```python
from build123d import *

# Parameters (mm, degrees)
F0_W     = 76
F0_H     = 70
F1_DEPTH = 3
F3_D     = 8.3
F4_SIZE  = 5


with BuildPart() as f1:
    # F0 (on Top) → F1 (new body)
    with BuildSketch(Plane.XY):
        Rectangle(F0_W, F0_H)
    extrude(amount=-F1_DEPTH)

    # F3 (through all)
    with Locations(Plane.XY):
        with Locations((-30, 25), (30, 25), (30, -25), (-30, -25)):
            Hole(F3_D / 2)

    # F4
    f4_edges = [f1.edges().sort_by_distance(p)[0] for p in [
        (-38, 35, -1.5),
        (-38, -35, -1.5),
        (38, -35, -1.5),
        (38, 35, -1.5),
    ]]
    chamfer(f4_edges, length=F4_SIZE)


solid = f1.part
```
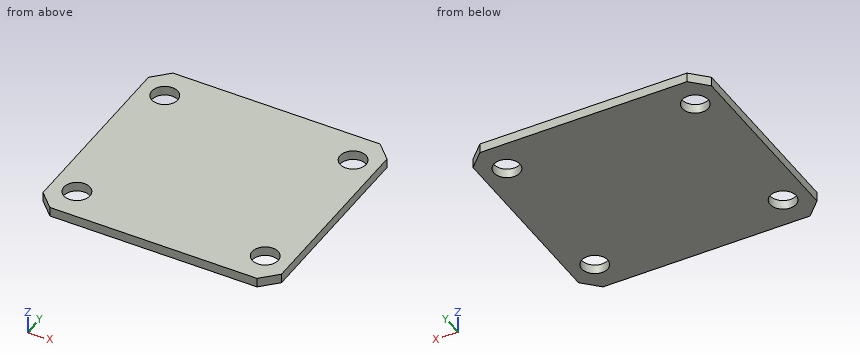
Geometry check sheet. Reference: the model listing, model coordinates, mm. Coordinates: 2 decimals unless noted, no trailing zeros. Order: outer loops, then holes, each group sorted by start corner. A loop starts at its lowest first (then second) coordinate and runs counter-clockwise, first axis right, second up. Notation, with made-up numbers: M 62.25,1 L 80.25,1 A23 cw 80.25,10 Z; hole C 9,-30 d3. An arc over 180 degrees is marked long. Answer as a JSON object with one key per item and string values.
Q1. Cross-section at C-C on x = -30. Record the cut outline in (y, z).
Results are:
{"outline": "M -35,-3 L -29.15,-3 L -29.15,0 L -35,0 Z; M -20.85,-3 L 20.85,-3 L 20.85,0 L -20.85,0 Z; M 29.15,-3 L 35,-3 L 35,0 L 29.15,0 Z"}
Q2. Cross-section at A-A on y = -25. Record the cut outline in (x, z), and give its area (3 significant figures).
Results are:
{"outline": "M -38,-3 L -34.15,-3 L -34.15,0 L -38,0 Z; M -25.85,-3 L 25.85,-3 L 25.85,0 L -25.85,0 Z; M 34.15,-3 L 38,-3 L 38,0 L 34.15,0 Z", "area": "178 mm²"}
Q3. Depth check by flat-ended pin: pin 1 Ø6.5 at (x, y) = (-30, 25) entering from +Z. Enter the tip coordinate at first touch or a pass-through.
Results are:
{"pin 1": "passes through"}
Q4. Scan lines: line 1 (Y direction, x = 30, z = -2.1); line 2 (X direction, y = -28, z = -2.35); line 3 (Y direction, x = -27, z = -0.2). Record each from-to range of solid material in increasing order.
Results are:
{"line 1": "y = -35 to -29.15, -20.85 to 20.85, 29.15 to 35", "line 2": "x = -38 to -32.87, -27.13 to 27.13, 32.87 to 38", "line 3": "y = -35 to -27.87, -22.13 to 22.13, 27.87 to 35"}
Q5. Cross-section at B-B on z = -1.05. Record the cut outline in (x, y), and give its area (3 significant figures).
Results are:
{"outline": "M -38,-30 L -33,-35 L 33,-35 L 38,-30 L 38,30 L 33,35 L -33,35 L -38,30 Z; hole C -30,-25 d8.3; hole C -30,25 d8.3; hole C 30,-25 d8.3; hole C 30,25 d8.3", "area": "5,050 mm²"}
